```python
from build123d import *

# Parameters (mm, degrees)
SKETCH_1_W      = 65
SKETCH_1_H      = 56
SKETCH_1_R      = 1.35
EXTRUDE_1_DEPTH = 15
SKETCH_2_W      = 85
SKETCH_2_H      = 56
EXTRUDE_2_DEPTH = 20


with BuildPart() as part:
    # 草图1 → 凸台-拉伸1 (new body)
    with BuildSketch(Plane.XY):
        Rectangle(SKETCH_1_W, SKETCH_1_H)
        with Locations((-29, 24.5)):
            Circle(SKETCH_1_R, mode=Mode.SUBTRACT)
        with Locations(Location((29, 24.5, 0), (0, 0, 180))):
            Circle(SKETCH_1_R, mode=Mode.SUBTRACT)
        with Locations(Location((-29, -24.5, 0), (0, 0, 180))):
            Circle(SKETCH_1_R, mode=Mode.SUBTRACT)
        with Locations((29, -24.5)):
            Circle(SKETCH_1_R, mode=Mode.SUBTRACT)
    extrude(amount=EXTRUDE_1_DEPTH)

    # 草图2 → 凸台-拉伸2 (add)
    with BuildSketch(Plane.XY.offset(15)):
        with Locations((10, 0)):
            Rectangle(SKETCH_2_W, SKETCH_2_H)
    extrude(amount=EXTRUDE_2_DEPTH)


solid = part.part
```
Verification items for the finished model (mm, model axes). A direction names the side the tool comes from. Give positions to 0.01 mm unless a question says otherwise; leave off trailing zeros. Loops run counter-clockwise (first coordinate to the right, second up) from the corner with the lowest first, then second, coordinate; pieces in that order, holes last. Notation, with made-up numbers: M -16,82 L 26,82 A28 cw 26,120 Z; hole C 41,24 d6. An arc over 180 degrees is marked long. Return JSON: item names as keys, results as strings.
1) Mould release check, pull along Y, two halves, no side actions. Record for faces 4 (the flat face through (9, 28, 17)), 5 (the flat face through (0, 0, 0)), 6 (the flat face through (-29, 25, 15)): released by +Y, released by -Y, zero draft, split by the parting line, or undercut.
Findings:
{"face 4": "released by +Y", "face 5": "zero draft", "face 6": "undercut"}
2) Section check B-B, the plane x = -29. Enter the section's corners in (y, z), and give its area (3 significant figures).
Findings:
{"outline": "M -28,0 L -25.85,0 L -25.85,15 L -23.15,15 L -23.15,0 L 23.15,0 L 23.15,15 L 25.85,15 L 25.85,0 L 28,0 L 28,35 L -28,35 Z", "area": "1,880 mm2"}
3) Section check C-C, the plane y = -24.5. Enter the section's corners in (x, z), and give its area (3 significant figures).
Findings:
{"outline": "M -32.5,0 L -30.35,0 L -30.35,15 L -27.65,15 L -27.65,0 L 27.65,0 L 27.65,15 L 30.35,15 L 30.35,0 L 32.5,0 L 32.5,15 L 52.5,15 L 52.5,35 L -32.5,35 Z", "area": "2,590 mm2"}
4) Gauge pin test, flat end, axial feed: P1, Ø1.4, axis at x = 29, y = 24, coming from the -Z side. Record the tip position at first contact, or that the pin passes through.
Findings:
{"P1": "stops at z = 15"}
5) Tool access check on faces 1 (the flat face through (29, -24, 15)), 2 (the flat face through (-32.5, 0, 17)), 3 (the flat face through (42, 0, 15)). Record the directions out of +Z, -Z, +X, -X, +Y, -Y that give a thin tool (end or side, any length) a straight path to the whole face; none if there is none.
Findings:
{"face 1": "-Z", "face 2": "+Z, -Z, -X, +Y, -Y", "face 3": "-Z, +X, +Y, -Y"}
6) Material ranges on L1, parallel to X at y = -24, z = 7; L2, parallel to Z at x = 36.5, y = 24.5; L3, parallel to X at y = -8.5, z = 3, recorded low to high. Write a range as [from, to].
Findings:
{"L1": "x = [-32.5, -30.25], [-27.75, 27.75], [30.25, 32.5]", "L2": "z = [15, 35]", "L3": "x = [-32.5, 32.5]"}
7) Section check D-D, the plane y = 4.5. Enter the section's corners in (x, z), and give its area (4 significant figures).
Findings:
{"outline": "M -32.5,0 L 32.5,0 L 32.5,15 L 52.5,15 L 52.5,35 L -32.5,35 Z", "area": "2,675 mm2"}
8) Section check A-A, the plane z = 11. Enter the section's corners in (x, y).
Findings:
{"outline": "M -32.5,-28 L 32.5,-28 L 32.5,28 L -32.5,28 Z; hole C -29,-24.5 d2.7; hole C -29,24.5 d2.7; hole C 29,-24.5 d2.7; hole C 29,24.5 d2.7"}
